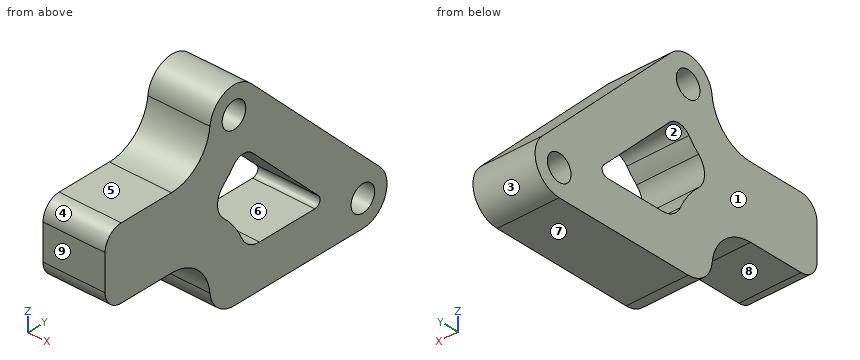
Autodesk Inventor part; units mm, degrees
ref_plane "YZ Plane" through (0, 0, 0) normal (1, 0, 0) x (0, 1, 0)
ref_plane "XZ Plane" through (0, 0, 0) normal (0, 1, 0) x (-1, 0, 0)
ref_plane "XY Plane" through (0, 0, 0) normal (0, 0, 1) x (1, 0, 0)
sketch "Sketch1" plane through (0, 0, 0) normal (1, 0, 0) x (0, 1, 0)
  line L0 (-12.6683, 12.8416) -> (-12.6683, 0.1416)
  line L1 (-12.6683, 0.1416) -> (-12.6683, -12.5584)
  line L2 (-12.6683, -12.5584) -> (0.0318, -12.5584)
  line L3 (0.0318, -12.5584) -> (12.7318, -12.5584)
  circle A0 centre (-12.6683, 12.8416) radius 2.3241
  circle A1 centre (12.7318, -12.5584) radius 2.3241
  line L4 (-12.6683, 12.8416) -> (-12.6683, -12.5584) construction
  line L5 (-17.4308, 12.8416) -> (-17.4308, -12.5584)
  line L6 (-7.9058, -12.5584) -> (-7.9058, 12.8416)
  arc A2 (-7.9058, 12.8416) -> (-17.4308, 12.8416) centre (-12.6683, 12.8416) ccw
  arc A3 (-17.4308, -12.5584) -> (-7.9058, -12.5584) centre (-12.6683, -12.5584) ccw
  line L7 (12.7318, -12.5584) -> (-12.6683, -12.5584) construction
  line L8 (12.7318, -7.7959) -> (-12.6683, -7.7959)
  line L9 (-12.6683, -17.3209) -> (12.7318, -17.3209)
  arc A4 (12.7318, -17.3209) -> (12.7318, -7.7959) centre (12.7318, -12.5584) ccw
  arc A5 (-12.6683, -7.7959) -> (-12.6683, -17.3209) centre (-12.6683, -12.5584) ccw
  line L10 (-12.6683, 0.1416) -> (-38.0683, 0.1416)
  arc A6 (-7.9058, 4.3417) -> (-7.9058, -4.0585) centre (-12.6683, 0.1416) ccw
  line L11 (-12.6683, 6.4916) -> (-34.8933, 6.4916)
  line L12 (-38.0683, 3.3166) -> (-38.0683, -3.0334)
  line L13 (-34.8933, -6.2084) -> (-12.6683, -6.2084)
  arc A7 (-34.8933, 6.4916) -> (-38.0683, 3.3166) centre (-34.8933, 3.3166) ccw
  arc A8 (-38.0683, -3.0334) -> (-34.8933, -6.2084) centre (-34.8933, -3.0334) ccw
  point P0 (0, 0)
  point P1 (0.0317, -12.5584)
  point P2 (-7.9058, -7.7959)
  point P3 (-17.4308, -6.2084)
  point P4 (-17.4308, 6.4916)
  dimension "d1" = 4.6482
  dimension "d2" = 4.6482
  dimension "d3" = 9.525
  dimension "d7" = 25.4
  dimension "d8" = 12.7
  dimension "d9" = 3.175
extrude "Extrusion1" add sketch "Sketch1" along normal blind 11.1125
fillet "Fillet1" radius 7.62 1 edges at (5.5563, -17.4308, -6.2084)
sketch "Sketch3" plane through (11.1125, 0, 0) normal (1, 0, 0) x (0, 0, -1)
  arc A0 (-12.8416, -7.9058) -> (-12.8416, -17.4308) centre (-12.8416, -12.6683) ccw
  line L0 (-12.8416, -17.4308) -> (-6.4916, -17.4308)
  line L1 (-6.4916, -17.4308) -> (-6.4916, -34.8933)
  arc A1 (-6.4916, -34.8933) -> (-3.3166, -38.0683) centre (-3.3166, -34.8933) ccw
  line L2 (-3.3166, -38.0683) -> (3.0334, -38.0683)
  arc A2 (3.0334, -38.0683) -> (6.2084, -34.8933) centre (3.0334, -34.8933) ccw
  line L3 (6.2084, -34.8933) -> (6.2084, -24.9854)
  arc A3 (13.0468, -17.4056) -> (6.2084, -24.9854) centre (13.8284, -24.9854) ccw
  arc A4 (13.0468, -17.4056) -> (17.3209, -12.6683) centre (12.5584, -12.6683) ccw
  line L4 (17.3209, -12.6683) -> (17.3209, 12.7318)
  arc A5 (17.3209, 12.7318) -> (7.7959, 12.7318) centre (12.5584, 12.7318) ccw
  line L5 (7.7959, 12.7318) -> (7.7959, -7.9058)
  line L6 (7.7959, -7.9058) -> (-12.8416, -7.9058)
  circle A6 centre (-12.8416, -12.6683) radius 2.3241
  circle A7 centre (12.5584, 12.7318) radius 2.3241
  line L7 (-16.2092, -9.3007) -> (9.1908, 16.0993)
  arc A8 (-12.8416, -7.9058) -> (-12.8416, -17.4308) centre (-12.8416, -12.6683) ccw
  point P0 (0, 0)
extrude "Extrusion2" add sketch "Sketch3" against normal up to surface (11.1125 mm away) contours A0 L7 A5 L5 L6
fillet "Fillet2" radius 7.62 1 edges at (5.5563, -17.4308, 6.4916)
sketch "Sketch4" plane through (11.1125, 0, 0) normal (1, 0, 0) x (0, 0, -1)
  arc A0 (-16.2092, -9.3007) -> (-13.3301, -17.4056) centre (-12.8416, -12.6683) ccw
  arc A1 (-6.4916, -24.9854) -> (-13.3301, -17.4056) centre (-14.1116, -24.9854) ccw
  line L0 (-6.4916, -24.9854) -> (-6.4916, -34.8933)
  arc A2 (-6.4916, -34.8933) -> (-3.3166, -38.0683) centre (-3.3166, -34.8933) ccw
  line L1 (-3.3166, -38.0683) -> (3.0334, -38.0683)
  arc A3 (3.0334, -38.0683) -> (6.2084, -34.8933) centre (3.0334, -34.8933) ccw
  line L2 (6.2084, -34.8933) -> (6.2084, -24.9854)
  arc A4 (13.0468, -17.4056) -> (6.2084, -24.9854) centre (13.8284, -24.9854) ccw
  arc A5 (13.0468, -17.4056) -> (17.3209, -12.6683) centre (12.5584, -12.6683) ccw
  line L3 (17.3209, -12.6683) -> (17.3209, 12.7318)
  arc A6 (17.3209, 12.7318) -> (9.1908, 16.0993) centre (12.5584, 12.7318) ccw
  line L4 (9.1908, 16.0993) -> (-16.2092, -9.3007)
  circle A7 centre (-12.8416, -12.6683) radius 2.3241
  circle A8 centre (12.5584, 12.7318) radius 2.3241
  arc A9 (-0.1416, -18.7795) -> (-7.3449, -11.2783) centre (-14.1116, -24.9854) ccw
  arc A10 (9.6545, -10.2799) -> (-0.1416, -18.7795) centre (13.8284, -24.9854) ccw
  line L5 (9.6545, -10.2799) -> (9.6545, 5.7211)
  line L6 (9.6545, 5.7211) -> (-7.3449, -11.2783)
  point P0 (0, 0)
extrude "Extrusion3" cut sketch "Sketch4" against normal blind 25.4 contours A9 L6 L5 A10
fillet "Fillet3" radius 3.81 1 edges at (5.5563, -10.2799, -9.6545)
fillet "Fillet4" radius 3.556 1 edges at (5.5563, -18.7795, 0.1416)
fillet "Fillet5" radius 2.54 1 edges at (5.5563, -11.2783, 7.3449)
fillet "Fillet6" radius 1.016 1 edges at (5.5563, 5.7211, -9.6545)
properties part number "MOGO Mech"
Part model, mm, in its own coordinate system. Face numbers are marked on the shaded views. A direction names the side the tool comes from. Round coordinates to 2 decimals unless told otherwise and drop trailing zeros. Write each loop counter-clockwise with the first axis right and the second up, starting at its lowest first coordinate (ties: lowest second). Pieces come first, ordered by that corner, then holes.
Item 1: Which spindle directions (+Z, -Z, +X, -X, +Y, -Y) get a long thin tool onto all of the face, cutting with end or side? Do the marked faces 5, 6, 7, 8 and 9. Say none if no direction does.
Results:
face 5: +Z, +X, -X, -Y
face 6: +X, -X
face 7: -Z, +X, -X, +Y, -Y
face 8: -Z, +X, -X, -Y
face 9: +Z, -Z, +X, -X, -Y
Item 2: Probe L1, parallel to Y at x = 9.25, z = 5.5; L2, parallel to Z at x = 1.5, y = -12.5; L3, parallel to Y at x = 8.25, z = 12. List the from-to ranges inside material, lowest first.
Results:
L1: y = -37.2 to -12.07, -9.56 to 1.41
L2: z = -17.32 to -5.01, 5.2 to 10.52, 15.16 to 17.6
L3: y = -17.66 to -14.83, -10.5 to -5.09
Item 3: Cut at C-C, the plane x = 8.25. Count the separate pieces of the cut face and the enclosed holes in it, plus the area to 3 significant figures.
Results:
separate pieces: 1
enclosed holes: 3
area: 880 mm2
Item 4: Cut at A-A, the plane y = -0.5. Give the cut face in (x, z), plus the area to 3 significant figures.
Results:
outline: (0, -17.32) - (11.11, -17.32) - (11.11, -9.65) - (0, -9.65) - close; (0, -3.43) - (11.11, -3.43) - (11.11, 7.41) - (0, 7.41) - close
area: 206 mm2
Item 5: Cut at B-B, the plane y = -30. Give the cut face in (x, z), plus the area to 3 significant figures.
Results:
outline: (0, -6.21) - (11.11, -6.21) - (11.11, 6.49) - (0, 6.49) - close
area: 141 mm2
Item 6: Drop flat-ended pins along their axis: pin 1 Ø1 at (y, z) = (-3, -2.5) entering from +X; pin 2 Ø3.5 at (x, y) = (5, -1.5) entering from +Z; pin 3 Ø3 at (x, y) = (7.5, -30.5) entering from +Z. Give the stop position or say it passes through.
Results:
pin 1: passes through
pin 2: stops at z = 10.16
pin 3: stops at z = 6.49
Item 7: Two-plate mould, pull along Y, no slides. Class the marked faces 1, 2, 3 and 4: +Y half, -Y half, draft (parallel to the pull), parting line (faces both ways), or undercut.
Results:
face 1: draft
face 2: undercut
face 3: +Y half
face 4: -Y half
